Can you work these out from the model? Positions are in its coordinate system, mm. Face numbers are marked on the shaded views. Round coordinates to 2 decimals unless told otherwise and drop trailing zeros. Order: outer loops, then holes, each group sorted by start corner. A loop starts at its lowest first (then second) coordinate and runs counter-clockwise, first axis right, second up. Notation, with made-up numbers: M -27.5,6 L 24.5,6 A25 ccw 24.5,44 Z; hole C 89,20.5 d6. An arc over 180 degrees is marked long. One line per question, with ' | ' between items.
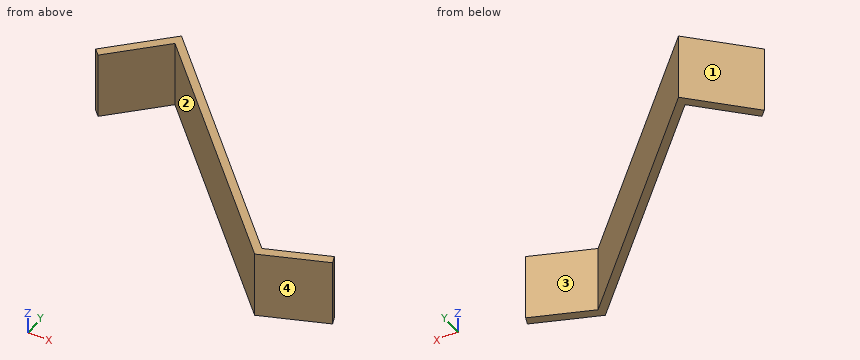
Autodesk Inventor part; units mm, degrees
ref_plane "YZ Plane" through (0, 0, 0) normal (1, 0, 0) x (0, 1, 0)
ref_plane "XZ Plane" through (0, 0, 0) normal (0, 1, 0) x (-1, 0, 0)
ref_plane "XY Plane" through (0, 0, 0) normal (0, 0, 1) x (1, 0, 0)
sketch "Sketch1" plane through (0, 0, 0) normal (0, 0, 1) x (1, 0, 0)
  line L0 (0, 0) -> (17.9605, 17.9605)
  line L1 (0, 0) -> (25.4, 0) construction
  line L2 (17.7799, 22.2704) -> (-2.2453, 2.2453)
  line L3 (-2.2453, 2.2453) -> (0, 0)
  line L4 (17.9605, 17.9605) -> (95.5858, -59.6648)
  line L5 (17.9605, 17.9605) -> (127.7393, 17.9605) construction
  line L6 (95.5858, -59.6648) -> (119.2185, -50.3557)
  line L7 (95.5858, -59.6648) -> (120.9858, -59.6648) construction
  line L8 (119.2185, -50.3557) -> (118.0548, -47.4016)
  line L9 (118.0548, -47.4016) -> (96.1001, -56.0498)
  line L10 (96.1001, -56.0498) -> (17.7799, 22.2704)
  dimension "d14" = 25.4
  dimension "d15" = 45
  dimension "d24" = 109.7788
  dimension "d25" = 45
  dimension "d26" = 25.4
  dimension "d27" = 21.5
  dimension "d28" = 3.175
  dimension "d29" = 23.5966
extrude "Extrusion2" add sketch "Sketch1" along normal blind 25.4
properties part number "LoadSlideBracket"
(1) Please list where these lines run through material, in increasing order: probe 1 along X at (y, z) = (13.5, 20.75); probe 2 along X at (y, z) = (-31, 17); probe 3 along Y at (x, z) = (80, 2). Write a range as [from, to].
Final values:
probe 1: [9.01, 13.5], [22.42, 26.55] | probe 2: [66.92, 71.05] | probe 3: [-44.08, -39.95]
(2) If we section it at B-B on y = 6: Please give me the cut outline in (x, z).
Final values:
outline: M 1.51,0 L 6,0 L 6,25.4 L 1.51,25.4 Z; M 29.92,0 L 34.05,0 L 34.05,25.4 L 29.92,25.4 Z
(3) Will these pins go through, and if not, where does the flat tip stop? pin 1 Ø1 at (x, z) = (75.5, 16.5) entering from -Y; pin 2 Ø12 at (y, z) = (-21, 7) entering from -X; pin 3 Ø8 at (x, y) = (18, 10) entering from -Z; pin 4 Ø10 at (y, z) = (-40.5, 17) entering from +X.
Final values:
pin 1: y = -40.08 | pin 2: x = 50.92 | pin 3: through | pin 4: x = 85.55
(4) Thinking about a two-plate mould opening in X: for the marked faces 1, 2, 3 and 4, which applies, released by +X, released by -X, zero draft, split by the parting line, or undercut?
Final values:
face 1: released by -X | face 2: undercut | face 3: undercut | face 4: released by +X
(5) If we section it at A-A on z = 4.75: Please give me the cut outline in (x, y), plus the area to 3 significant figures.
Final values:
outline: M -2.25,2.25 L 0,0 L 17.96,17.96 L 95.59,-59.66 L 119.22,-50.36 L 118.05,-47.4 L 96.1,-56.05 L 17.78,22.27 Z | area: 485 mm^2
(6) If we section it at C-C on x = 69.5: Please give me the cut outline in (y, z), plus the area to 3 significant figures.
Final values:
outline: M -33.58,0 L -29.45,0 L -29.45,25.4 L -33.58,25.4 Z | area: 105 mm^2
(7) If we section it at D-D on y = -21: Please give me the cut outline in (x, z).
Final values:
outline: M 56.92,0 L 61.05,0 L 61.05,25.4 L 56.92,25.4 Z
